The listing builds one solid part. Answer for the finished solid, in the listing's coordinates (mm). Face numbers are marked on the shaded views. A direction names the side the tool comes from. Round coordinates to 2 decimals unless told otherwise and drop trailing zeros. Write each loop counter-clockwise with the first axis right and the second up, starting at its lowest first coordinate (ties: lowest second). Pieces come first, ordered by that corner, then holes.
Item 1: Find section A-A on x = 0. Give the vertices of the cut face in (y, z).
Item 2: A tool of negligible diameter and unlimited length cuts with its end or side. For the marked faces 1 and 2, from which of +Z, -Z, +X, -X, +Y, -Y can it reach the whole face along a straight path? Write none if from no direction.
Item 3: Find section B-B on y = -3.5. Give the vertices of the cut face in (x, z).
Item 4: Find section C-C on y = -7.5. Give the vertices of the cut face in (x, z), then the cut area to 3 significant figures.
Item 5: Each of these flat-tipped pins is pushed along its axis until it touches: pin 1 (1.5 mm diameter, centred on y = -3.5, z = 1, fed in from +X); pin 2 (4 mm diameter, centred on y = -13, z = 0, fed in from -X); pin 3 (2 mm diameter, centred on x = 1, y = -18.5, fed in from -Z). Where does it stop, or does it pass through?
Item 6: Find section D-D on x = 6.75. Give the vertices of the cut face in (y, z), then the cut area to 3 significant figures.
Item 7: Find the intervals of material crossed by probe 1 along Y at (x, z) = (-1.25, 6.75); probe 2 along X at (y, z) = (-5.75, -2.5); probe 3 along X at (y, z) = (-2.5, -2.75), in increasing order.
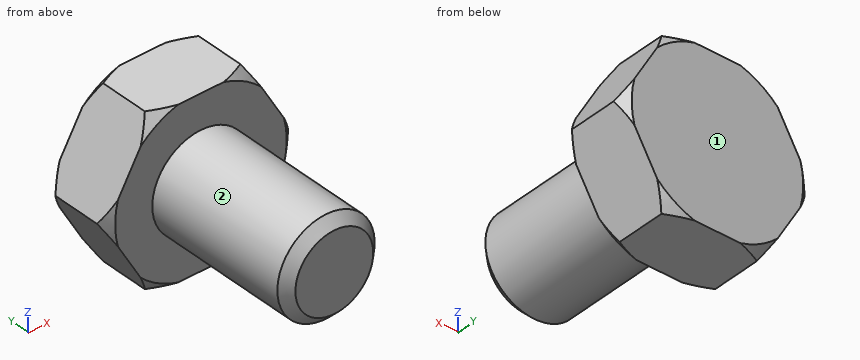
```python
from build123d import *

# Parameters (mm, degrees)
EXTRUDE_1_DEPTH = 7
SKETCH_5_R      = 5
EXTRUDE_2_DEPTH = 16
CHAMFER_1_SIZE  = 1


with BuildPart() as part:
    # Эскиз1 → Вытянуть1 (new body)
    with BuildSketch(Plane(origin=(0, 0, 0), x_dir=(1, 0, 0), z_dir=(0, 1, 0))):
        Polygon((-9.814954576, 0), (-4.907477288, 8.5), (4.907477288, 8.5), (9.814954576, 0), align=None)
        Polygon((-9.814954576, 0), (9.814954576, 0), (4.907477288, -8.5), (-4.907477288, -8.5), align=None)
    extrude(amount=-EXTRUDE_1_DEPTH)

    # Эскиз5 → Вытянуть2 (add)
    with BuildSketch(Plane.XZ.offset(7)):
        with Locations(Location((0, 0, 0), (0, 0, 90))):
            Circle(SKETCH_5_R)
    extrude(amount=EXTRUDE_2_DEPTH)

    # Эскиз4 → Вырез-Повернуть1 (revolve, cut)
    with BuildSketch(Plane.XY):
        Polygon((-9.814954576, -1), (-8.814954576, 0), (-9.814954576, 0), align=None)
        Polygon((-9.814954576, -6), (-8.814954576, -7), (-9.814954576, -7), align=None)
    revolve(axis=Axis((0, -7, 0), (0, -1, 0)), mode=Mode.SUBTRACT)

    # Фаска1
    chamfer_1_edges = [part.edges().sort_by_distance(p)[0] for p in [
        (0, -23, -5),
    ]]
    chamfer(chamfer_1_edges, length=CHAMFER_1_SIZE)


solid = part.part
```
Check values:
1. outline: (-23, -4) - (-22, -5) - (-7, -5) - (-7, -8.5) - (0, -8.5) - (0, 8.5) - (-7, 8.5) - (-7, 5) - (-22, 5) - (-23, 4) - close
2. face 1: +Z, -Z, +X, -X, +Y
2. face 2: -Y
3. outline: (-9.81, 0) - (-4.91, -8.5) - (4.91, -8.5) - (9.81, 0) - (4.91, 8.5) - (-4.91, 8.5) - close
4. outline: circle Ø10 at (0, 0)
4. area: 78.5 mm2
5. pin 1: stops at x = 9.67
5. pin 2: stops at x = -5
5. pin 3: stops at z = -5
6. outline: (-7, -5.31) - (0, -5.31) - (0, 5.31) - (-7, 5.31) - close
6. area: 74.3 mm2
7. probe 1: y = -7 to 0
7. probe 2: x = -8.37 to 8.37
7. probe 3: x = -8.23 to 8.23
